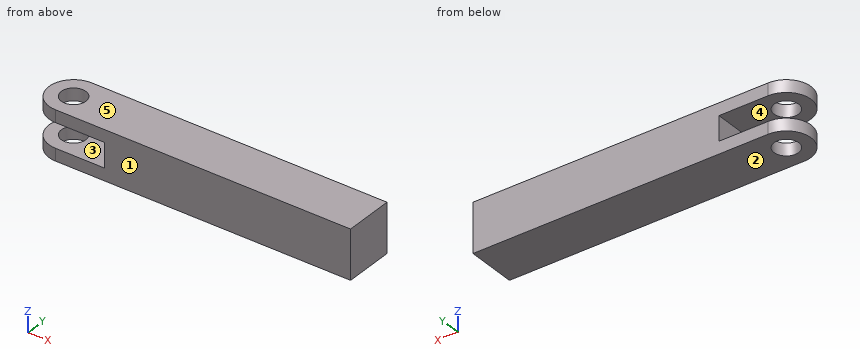
```python
from build123d import *

# Parameters (mm, degrees)
SKETCH_1_W      = 50
SKETCH_1_H      = 10
EXTRUDE_1_DEPTH = 5
SKETCH_2_R      = 2.5
EXTRUDE_2_DEPTH = 2.5


with BuildPart() as part:
    # 草图1 → 凸台-拉伸1 (new, symmetric)
    with BuildSketch(Plane.XY):
        Rectangle(SKETCH_1_W, SKETCH_1_H)
    extrude(amount=EXTRUDE_1_DEPTH, both=True)

    # 草图2 → 凸台-拉伸2 (add)
    with BuildSketch(Plane(origin=(0, 0, -5), x_dir=(-1, 0, 0), z_dir=(0, 0, -1))):
        with BuildLine():
            Line((25, 5), (35, 5))
            ThreePointArc((35, 5), (40, 0), (35, -5))
            Line((35, -5), (25, -5))
            Line((25, -5), (25, 5))
        make_face()
        with Locations((35, 0)):
            Circle(SKETCH_2_R, mode=Mode.SUBTRACT)
    extrude_2 = extrude(amount=-EXTRUDE_2_DEPTH)

    # 镜向1: 凸台-拉伸2 across plane
    add(extrude_2.mirror(Plane.XY))


solid = part.part
```
Could you check a few things on this model? Use its own coordinates, in mm. Face numbers are marked on the shaded views. A direction names the side the tool comes from. Round coordinates to 2 decimals unless told otherwise and drop trailing zeros. Loops run counter-clockwise (first coordinate to the right, second up) from the corner with the lowest first, then second, coordinate; pieces in that order, holes last. Notation, with made-up numbers: M -19.5,-22.75 L 31.5,-22.75 A28 cw 31.5,5.25 Z; hole C -25,39 d11. An arc over 180 degrees is marked long. Write item = value, one per line.
1. I want a section at B-B, the plane x = -34. Write out the boundary of the cut face in (y, z).
Results below:
outline = M -5,-5 L -2.29,-5 L -2.29,-2.5 L -5,-2.5 Z; M -5,2.5 L -2.29,2.5 L -2.29,5 L -5,5 Z; M 2.29,-5 L 5,-5 L 5,-2.5 L 2.29,-2.5 Z; M 2.29,2.5 L 5,2.5 L 5,5 L 2.29,5 Z
2. I want a section at C-C, the plane z = -4.25. Write out the boundary of the cut face in (x, y), and give its area (3 significant figures).
Results below:
outline = M -35,-5 L 25,-5 L 25,5 L -35,5 A5 ccw Z; hole C -35,0 d5
area = 620 mm²
3. Thinking about a two-plate mould opening in Z: for the marked faces 1, 2 and 3, which applies, +Z half, -Z half, draft (parallel to the pull), parting line (faces both ways), or undercut?
Results below:
face_1 = draft
face_2 = -Z half
face_3 = undercut
4. Which directions (+Z, -Z, +X, -X, +Y, -Y) give clear straight access to the entire face, cutting with the end or side of a thin tool? Please do the marked faces 4 and 5.
Results below:
face_4 = -X, +Y, -Y
face_5 = +Z, +X, -X, +Y, -Y
5. I want a section at A-A, the plane y = 0. Write out the boundary of the cut face in (x, z).
Results below:
outline = M -40,-5 L -37.5,-5 L -37.5,-2.5 L -40,-2.5 Z; M -40,2.5 L -37.5,2.5 L -37.5,5 L -40,5 Z; M -32.5,-5 L 25,-5 L 25,5 L -32.5,5 L -32.5,2.5 L -25,2.5 L -25,-2.5 L -32.5,-2.5 Z
6. I want a section at D-D, the plane y = 3.75. Write out the boundary of the cut face in (x, z).
Results below:
outline = M -38.31,-5 L 25,-5 L 25,5 L -38.31,5 L -38.31,2.5 L -25,2.5 L -25,-2.5 L -38.31,-2.5 Z
7. Will this pin go through, and if not, where does the flat tip stop? P1, Ø1.5, axis at y = -3, z = -3.5, coming from the -X side.
Results below:
P1 = -39.47
8. I need wall thicknesses on probe 1 along Z at (x, y) = (-33.5, 3.5); probe 2 along X at (y, z) = (2, -1.75). Which ranges of each line are inside material? Lowest first, please.
Results below:
probe_1 = -5 to -2.5, 2.5 to 5
probe_2 = -25 to 25
